Geometry check sheet. Reference: the model listing, model coordinates, mm. A direction names the side the tool comes from. Round coordinates to 2 decimals unless told otherwise and drop trailing zeros. Order: outer loops, then holes, each group sorted by start corner. A loop starts at its lowest first (then second) coordinate and runs counter-clockwise, first axis right, second up.
(1) Draft check along X on faces 3 (the face through (6, -7, -27)), 4 (the face through (-20.582, -4, -33)), 5 (the face through (5, -15.85, -33)). Enter one of: pulls with the +X half, pulls with the -X half, needs draft (parallel to the pull), parting line crosses it, or undercut.
(2) Cross-section at C-C on x = 8. Enter the section's corners in (y, z), and give its area (3 significant figures).
(3) Thickness scan on L1, parallel to X at y = -5.5, z = -24; L2, parallel to X at y = -5, z = -41; L3, parallel to Y at x = -2, z = -10. Record the ranges inside material, lowest first.
(4) Cross-section at B-B on z = -12. Enter the section's corners in (x, y), and give its area (3 significant figures).
(5) Set-up check for faces 1 (the face through (5, -12, 0)), 2 (the face through (3.983, -11.645, -13.311)): record each of +Z, -Z, +X, -X, +Y, -Y from which the full face is reachable in a straight line by a thin tool's end or side.
(6) Cross-section at D-D on y = -10.75. Enter the section's corners in (x, z).
(7) Cross-section at A-A on y = 5. Enter the section's corners in (x, z).
(8) Gauge pin test, flat ends, axial feed: P1, Ø1.5, axis at x = -2.5, z = -7, coming from the +Y side; P2, Ø3, axis at x = -10, y = -2.5, coming from the +Z side. Record the tip position at first contact, or that the pin passes through.
from build123d import *

# Parameters (mm, degrees)
BOSS_EXTRUDE1_DEPTH = 66.5
SKETCH4_R           = 19.8
CUT_EXTRUDE1_DEPTH  = 27
SKETCH5_R           = 15
CUT_EXTRUDE2_DEPTH  = 52.738521814


with BuildPart() as part:
    # Sketch1 → Boss-Extrude1 (new body)
    with BuildSketch(Plane.XY):
        Polygon((-20.582022726, -5.70241059), (-20.582022726, 8.150480999), (29.417977274, 8.150480999), (29.417977274, -11.649519001), (29.417977274, -15.849519001), (-20.582022726, -15.849519001), align=None)
    extrude(amount=-BOSS_EXTRUDE1_DEPTH)

    # Sketch4 → Cut-Extrude1 (cut)
    with BuildSketch(Plane.XY):
        with Locations((4.417977274, 8.150480999)):
            Circle(SKETCH4_R)
    extrude(amount=-CUT_EXTRUDE1_DEPTH, mode=Mode.SUBTRACT)

    # Sketch5 → Cut-Extrude2 (cut, through all)
    with BuildSketch(Plane.XY.offset(-27)):
        with Locations((4.417977274, 8.150480999)):
            Circle(SKETCH5_R)
    extrude(amount=-CUT_EXTRUDE2_DEPTH, mode=Mode.SUBTRACT)


solid = part.part
Found:
1. face 3: undercut
1. face 4: pulls with the -X half
1. face 5: needs draft
2. outline: (-15.85, -66.5) - (-6.42, -66.5) - (-6.42, -27) - (-11.32, -27) - (-11.32, 0) - (-15.85, 0) - close
2. area: 495 mm2
3. L1: x = -20.58 to -9.92, 18.76 to 29.42
3. L2: x = -20.58 to -2.8, 11.63 to 29.42
3. L3: y = -15.85 to -10.58
4. outline: (-20.58, -15.85) - (29.42, -15.85) - (29.42, 8.15) - (24.22, 8.15) arc R19.8 cw to (-15.38, 8.15) - (-20.58, 8.15) - close
4. area: 584 mm2
5. face 1: +Z, +X, -X, +Y, -Y
5. face 2: +Z, +Y
6. outline: (-20.58, -66.5) - (29.42, -66.5) - (29.42, 0) - (10.32, 0) - (10.32, -27) - (-1.48, -27) - (-1.48, 0) - (-20.58, 0) - close
7. outline: (-20.58, -66.5) - (-10.25, -66.5) - (-10.25, -27) - (-15.13, -27) - (-15.13, 0) - (-20.58, 0) - close; (19.08, -66.5) - (29.42, -66.5) - (29.42, 0) - (23.97, 0) - (23.97, -27) - (19.08, -27) - close
8. P1: stops at y = -10.1
8. P2: stops at z = -27
